Can you work these out from the drawing? Everything is in mm from the part's minimum corner. A direction names the side the tool comes from. Round coordinates to 2 decimals unless told otherwise and drop trailing zeros. Order: outer loops, then holes, each group sorted by start corner. A loop starts at its lowest first (then second) coordinate and runs counter-clockwise, first axis right, second up. Notation, with made-up numbers: (-22.5, -16.5) -> (-16.5, -16.5) arc R23 cw to (-16.5, 16.5) -> close; hole circle Ø3 at (33.5, 26). An arc over 180 degrees is marked (long way). One line per item, written item: value.
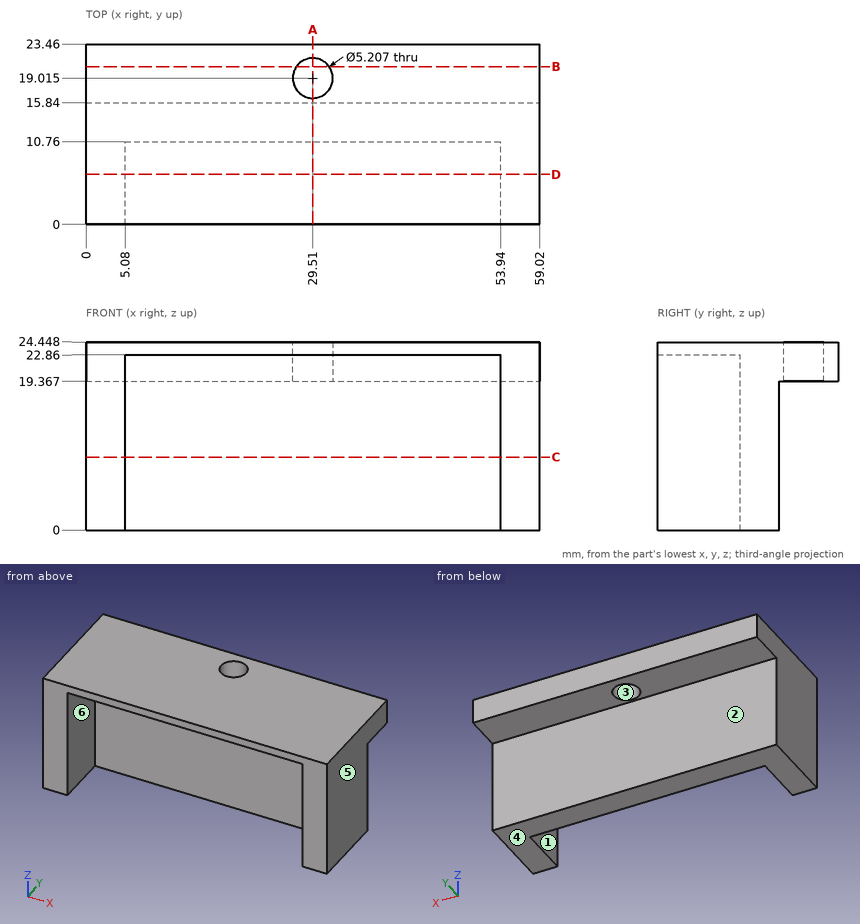
Q1. If we mould it in two halves opening along X, with no side actions, what happens to the marked faces 4, 5 and 6? For each: pulls with the +X half, pulls with the -X half, needs draft (parallel to the pull), parting line crosses it, or undercut.
Answers:
face 4: needs draft
face 5: pulls with the +X half
face 6: undercut
Q2. I need wall thicknesses on line 1 along X through (y, z) = (7.5, 11.5); line 2 along Y through (x, z) = (29.51, 21.15); line 3 along Z through (x, y) = (22, 21.25). Which ranges of each line are inside material? Lowest first, please.
Answers:
line 1: 0 to 5.08, 53.94 to 59.02
line 2: 10.76 to 16.41, 21.62 to 23.46
line 3: 19.37 to 24.45
Q3. Which directions (+Z, -Z, +X, -X, +Y, -Y) give clear straight access to the entire face, cutting with the end or side of a thin tool? Please do the marked faces 1, 2 and 3.
Answers:
face 1: -Z, -Y
face 2: -Z, +X, -X, +Y
face 3: +Z, -Z
Q4. For P1, Ø1.5, axis at x = 15, z = 16.5, coming from the +Y side; P2, Ø2.5, axis at x = 15, y = 18.5, coming from the -Z side; P3, Ø10, axis at x = 36.5, z = 4, coming from the -Y side, each with a flat end and sliding along its axis, tell me the tip position at first contact or that it passes through.
Answers:
P1: y = 15.84
P2: z = 19.37
P3: y = 10.76
Q5. I want a section at C-C on z = 9.5. Write out the boundary of the cut face in (x, y), then the cut area to 3 significant figures.
Answers:
outline: (0, 0) -> (5.08, 0) -> (5.08, 10.76) -> (53.94, 10.76) -> (53.94, 0) -> (59.02, 0) -> (59.02, 15.84) -> (0, 15.84) -> close
area: 409 mm2
Q6. I want a section at B-B on y = 20.5. Write out the boundary of the cut face in (x, z).
Answers:
outline: (0, 19.37) -> (27.37, 19.37) -> (27.37, 24.45) -> (0, 24.45) -> close; (31.65, 19.37) -> (59.02, 19.37) -> (59.02, 24.45) -> (31.65, 24.45) -> close
Q7. I want a section at D-D on y = 6.5. Write out the boundary of the cut face in (x, z).
Answers:
outline: (0, 0) -> (5.08, 0) -> (5.08, 22.86) -> (53.94, 22.86) -> (53.94, 0) -> (59.02, 0) -> (59.02, 24.45) -> (0, 24.45) -> close
Q8. I want a section at A-A on x = 29.51. Write out the boundary of the cut face in (y, z).
Answers:
outline: (0, 22.86) -> (10.76, 22.86) -> (10.76, 0) -> (15.84, 0) -> (15.84, 19.37) -> (16.41, 19.37) -> (16.41, 24.45) -> (0, 24.45) -> close; (21.62, 19.37) -> (23.46, 19.37) -> (23.46, 24.45) -> (21.62, 24.45) -> close
